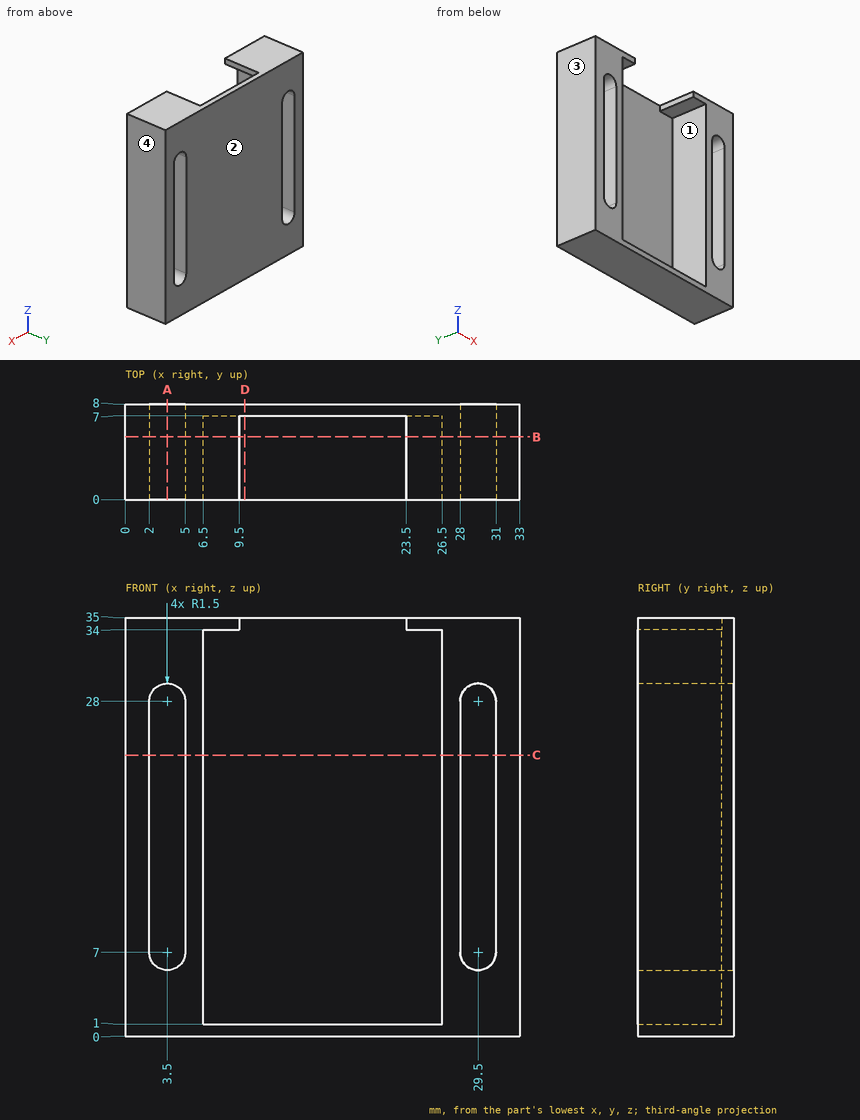
Check sheet for the drawn part. Datum: minimum x, y, z corner. Units: mm. Give positions to 0.01 mm unless a question says otherwise; leave off trailing zeros. Order: outer loops, then holes, each group sorted by start corner. A loop starts at its lowest first (then second) coordinate and runs counter-clockwise, first axis right, second up.
1. Scan lines: line 1 (X direction, y = 4.25, z = 22); line 2 (X direction, y = 7.5, z = 22); line 3 (X direction, y = 4.5, z = 3). Record each from-to range of solid material in increasing order.
Completed:
line 1: x = 0 to 2, 5 to 6.5, 26.5 to 28, 31 to 33
line 2: x = 0 to 2, 5 to 28, 31 to 33
line 3: x = 0 to 6.5, 26.5 to 33
2. Sectioned sample at A-A (x = 3.5). Record the boundary of the cut face in (y, z).
Completed:
outline: (0, 0) - (8, 0) - (8, 5.5) - (0, 5.5) - close; (0, 29.5) - (8, 29.5) - (8, 35) - (0, 35) - close
3. Depth check by flat-ended pin: pin 1 (2 mm diameter, centred on x = 18, y = 3, fed in from +Z); pin 2 (6 mm diameter, centred on x = 16.5, z = 11, fed in from -Y). Enter the tip coordinate at first touch or a pass-through.
Completed:
pin 1: stops at z = 1
pin 2: stops at y = 7
4. Sectioned sample at D-D (x = 10). Record the boundary of the cut face in (y, z).
Completed:
outline: (0, 0) - (8, 0) - (8, 35) - (7, 35) - (7, 1) - (0, 1) - close
5. Sectioned sample at C-C (z = 23.5). Record the boundary of the cut face in (x, y).
Completed:
outline: (0, 0) - (2, 0) - (2, 8) - (0, 8) - close; (5, 0) - (6.5, 0) - (6.5, 7) - (26.5, 7) - (26.5, 0) - (28, 0) - (28, 8) - (5, 8) - close; (31, 0) - (33, 0) - (33, 8) - (31, 8) - close
6. Draft check along X on the marked faces 1, 2, 3 and 4. Enter one of: pulls with the +X half, pulls with the -X half, needs draft (parallel to the pull), parting line crosses it, or undercut.
Completed:
face 1: undercut
face 2: needs draft
face 3: pulls with the -X half
face 4: pulls with the +X half
7. Sectioned sample at B-B (y = 5.25). Record the boundary of the cut face in (x, z), then the cut area to 3 significant figures.
Completed:
outline: (0, 0) - (33, 0) - (33, 35) - (23.5, 35) - (23.5, 34) - (26.5, 34) - (26.5, 1) - (6.5, 1) - (6.5, 34) - (9.5, 34) - (9.5, 35) - (0, 35) - close; hole (2, 7) arc R1.5 ccw to (5, 7) - (5, 28) arc R1.5 ccw to (2, 28) - close; hole (28, 7) arc R1.5 ccw to (31, 7) - (31, 28) arc R1.5 ccw to (28, 28) - close
area: 341 mm2
